```python
from build123d import *

# Parameters (mm, degrees)
SKETCH1_W               = 122
SKETCH1_H               = 185
BOSS_EXTRUDE1_DEPTH     = 20
CUT_EXTRUDE1_DEPTH      = 196.821347151
CUT_EXTRUDE2_REACH      = 156.403
CUT_EXTRUDE2_END_RADIUS = 7.5
SKETCH2_R               = 7.5


with BuildPart() as part:
    # Sketch1 → Boss-Extrude1 (new body)
    with BuildSketch(Plane(origin=(0, 0, 0), x_dir=(1, 0, 0), z_dir=(0, 1, 0))):
        Rectangle(SKETCH1_W, SKETCH1_H)
    extrude(amount=BOSS_EXTRUDE1_DEPTH)

    # Sketch3 → Cut-Extrude1 (cut, through all)
    with BuildSketch(Plane.XY.offset(92.5)):
        with BuildLine():
            Line((-50, 17.5), (50, 17.5))
            ThreePointArc((50, 17.5), (57.5, 10), (50, 2.5))
            Line((50, 2.5), (-50, 2.5))
            ThreePointArc((-50, 2.5), (-57.5, 10), (-50, 17.5))
        make_face()
    extrude(amount=-CUT_EXTRUDE1_DEPTH, mode=Mode.SUBTRACT)

    # Cut-Extrude2: up to this cylinder (the profile starts outside it)
    cut_extrude2_end = Plane(origin=(50, 10, 0), z_dir=(0, 0, 1)) * Cylinder(CUT_EXTRUDE2_END_RADIUS, 478.806, mode=Mode.PRIVATE)
    # Sketch2 → Cut-Extrude2 (cut, up to the surface)
    with BuildSketch(Plane(origin=(61, 0, 0), x_dir=(0, 0, -1), z_dir=(1, 0, 0)), mode=Mode.PRIVATE) as cut_extrude2_sk1:
        with Locations((-75, 10)):
            Circle(SKETCH2_R)
    cut_extrude2_tool1 = extrude(cut_extrude2_sk1.sketch, amount=-CUT_EXTRUDE2_REACH, mode=Mode.PRIVATE) - cut_extrude2_end
    add(cut_extrude2_tool1.solids().sort_by_distance((61, 10, 75))[0], mode=Mode.SUBTRACT)
    # Sketch2 → Cut-Extrude2 (cut, up to the surface)
    with BuildSketch(Plane(origin=(61, 0, 0), x_dir=(0, 0, -1), z_dir=(1, 0, 0)), mode=Mode.PRIVATE) as cut_extrude2_sk2:
        with Locations((-50, 10)):
            Circle(SKETCH2_R)
    cut_extrude2_tool2 = extrude(cut_extrude2_sk2.sketch, amount=-CUT_EXTRUDE2_REACH, mode=Mode.PRIVATE) - cut_extrude2_end
    add(cut_extrude2_tool2.solids().sort_by_distance((61, 10, 50))[0], mode=Mode.SUBTRACT)
    # Sketch2 → Cut-Extrude2 (cut, up to the surface)
    with BuildSketch(Plane(origin=(61, 0, 0), x_dir=(0, 0, -1), z_dir=(1, 0, 0)), mode=Mode.PRIVATE) as cut_extrude2_sk3:
        with Locations((-25, 10)):
            Circle(SKETCH2_R)
    cut_extrude2_tool3 = extrude(cut_extrude2_sk3.sketch, amount=-CUT_EXTRUDE2_REACH, mode=Mode.PRIVATE) - cut_extrude2_end
    add(cut_extrude2_tool3.solids().sort_by_distance((61, 10, 25))[0], mode=Mode.SUBTRACT)
    # Sketch2 → Cut-Extrude2 (cut, up to the surface)
    with BuildSketch(Plane(origin=(61, 0, 0), x_dir=(0, 0, -1), z_dir=(1, 0, 0)), mode=Mode.PRIVATE) as cut_extrude2_sk4:
        with Locations((0, 10)):
            Circle(SKETCH2_R)
    cut_extrude2_tool4 = extrude(cut_extrude2_sk4.sketch, amount=-CUT_EXTRUDE2_REACH, mode=Mode.PRIVATE) - cut_extrude2_end
    add(cut_extrude2_tool4.solids().sort_by_distance((61, 10, 0))[0], mode=Mode.SUBTRACT)
    # Sketch2 → Cut-Extrude2 (cut, up to the surface)
    with BuildSketch(Plane(origin=(61, 0, 0), x_dir=(0, 0, -1), z_dir=(1, 0, 0)), mode=Mode.PRIVATE) as cut_extrude2_sk5:
        with Locations((25, 10)):
            Circle(SKETCH2_R)
    cut_extrude2_tool5 = extrude(cut_extrude2_sk5.sketch, amount=-CUT_EXTRUDE2_REACH, mode=Mode.PRIVATE) - cut_extrude2_end
    add(cut_extrude2_tool5.solids().sort_by_distance((61, 10, -25))[0], mode=Mode.SUBTRACT)
    # Sketch2 → Cut-Extrude2 (cut, up to the surface)
    with BuildSketch(Plane(origin=(61, 0, 0), x_dir=(0, 0, -1), z_dir=(1, 0, 0)), mode=Mode.PRIVATE) as cut_extrude2_sk6:
        with Locations((50, 10)):
            Circle(SKETCH2_R)
    cut_extrude2_tool6 = extrude(cut_extrude2_sk6.sketch, amount=-CUT_EXTRUDE2_REACH, mode=Mode.PRIVATE) - cut_extrude2_end
    add(cut_extrude2_tool6.solids().sort_by_distance((61, 10, -50))[0], mode=Mode.SUBTRACT)
    # Sketch2 → Cut-Extrude2 (cut, up to the surface)
    with BuildSketch(Plane(origin=(61, 0, 0), x_dir=(0, 0, -1), z_dir=(1, 0, 0)), mode=Mode.PRIVATE) as cut_extrude2_sk7:
        with Locations((75, 10)):
            Circle(SKETCH2_R)
    cut_extrude2_tool7 = extrude(cut_extrude2_sk7.sketch, amount=-CUT_EXTRUDE2_REACH, mode=Mode.PRIVATE) - cut_extrude2_end
    add(cut_extrude2_tool7.solids().sort_by_distance((61, 10, -75))[0], mode=Mode.SUBTRACT)


solid = part.part
```
Here's how the part is built. I have some questions about the finished solid (model axes, mm). A direction names the side the tool comes from. Round coordinates to 2 decimals unless told otherwise and drop trailing zeros. Order: outer loops, then holes, each group sorted by start corner. A loop starts at its lowest first (then second) coordinate and runs counter-clockwise, first axis right, second up. Notation, with made-up numbers: M 51.25,-11 L 57.25,-11 A19 cw 57.25,17 Z; hole C 19.5,39.5 d3. An arc over 180 degrees is marked long. Use CSV: the item, a comma, the result in double quotes.
1) I want a section at A-A (x = -43). List the corners of the cut face in (y, z) for me, then the cut area to 3 significant figures.
Taken from the geometry:
outline,"M 0,-92.5 L 2.5,-92.5 L 2.5,92.5 L 0,92.5 Z; M 17.5,-92.5 L 20,-92.5 L 20,92.5 L 17.5,92.5 Z"
area,"925 mm^2"
2) On a 3-axis mill with a long thin cutter (end or side, diameter ignored), from which of +Z, -Z, +X, -X, +Y, -Y can I reach the whole of each face in a straight line? I mean faces 4 (the cylindrical face through (57.5, 10.16, 62.68)), 5 (the flat face through (0, 2, -92.5)), 6 (the cylindrical face through (58, 15.1, 30.5)). Say none if no direction works.
Taken from the geometry:
face 4,"+Z, -Z"
face 5,"-Z, +X, -X, +Y, -Y"
face 6,"+X"
3) I want a section at B-B (z = 11.5). List the corners of the cut face in (x, y) for me, then the cut area to 3 significant figures.
Taken from the geometry:
outline,"M -61,0 L 61,0 L 61,20 L -61,20 Z; hole M -50,2.5 L 50,2.5 A7.5 ccw 50,17.5 L -50,17.5 A7.5 ccw Z"
area,"763 mm^2"
4) I want a section at D-D (z = 44.5). List the corners of the cut face in (x, y) for me.
Taken from the geometry:
outline,"M -61,0 L 61,0 L 61,4.9 L 55.5,4.9 A7.5 cw 50,2.5 L -50,2.5 A7.5 cw -50,17.5 L 50,17.5 A7.5 cw 55.5,15.1 L 61,15.1 L 61,20 L -61,20 Z"
5) If we mould it in two halves opening along Z, with no side actions, what happens to faces 1 (the cylindrical face through (57.5, 10.16, -85.57)), 2 (the flat face through (0, 2, 92.5)), 3 (the cylindrical face through (58, 15.1, 80.5))? For each: pulls with the +Z half, pulls with the -Z half, needs draft (parallel to the pull), parting line crosses it, or undercut.
Taken from the geometry:
face 1,"needs draft"
face 2,"pulls with the +Z half"
face 3,"undercut"
6) I need wall thicknesses on line 1 along Y through (x, z) = (55.75, -50); line 2 along X through (y, z) = (9.25, -12.5); line 3 along Y through (x, z) = (52, 82). Which ranges of each line are inside material? Lowest first, please. Write a range as [from, to].
Taken from the geometry:
line 1,"[0, 2.5], [17.5, 20]"
line 2,"[-61, -57.46], [57.46, 61]"
line 3,"[0, 2.77], [17.23, 20]"
7) I want a section at C-C (z = -27.5). List the corners of the cut face in (x, y) for me.
Taken from the geometry:
outline,"M -61,0 L 61,0 L 61,2.93 L 52.5,2.93 A7.5 cw 50,2.5 L -50,2.5 A7.5 cw -50,17.5 L 50,17.5 A7.5 cw 52.5,17.07 L 61,17.07 L 61,20 L -61,20 Z"
8) I'm going to push flat-ended pins straight in: P1, Ø12, axis at y = 10, z = -25, coming from the +X side; P2, Ø8, axis at x = -41.5, y = 12, coming from the +Z side. Where does each tip first touch, or does it pass through?
Taken from the geometry:
P1,"x = -54.5"
P2,"through"
